from build123d import *

# Parameters (mm, degrees)
SHELL1_T           = -3
SKETCH2_R          = 35
CUT_EXTRUDE1_DEPTH = 131.048068171
SKETCH3_W          = 75
SKETCH3_H          = 50
CUT_EXTRUDE2_DEPTH = 131.048068171


with BuildPart() as part:
    # Sketch1 → Revolve1 (revolve)
    with BuildSketch(Plane.XY, mode=Mode.PRIVATE) as revolve1_sk:
        with BuildLine():
            Line((0, 40), (0, 0))
            Line((0, 0), (-87.5, 0))
            Line((-87.5, 0), (-87.5, 5))
            ThreePointArc((-87.5, 5), (-84.085301316, 16.215125476), (-75, 23.624343151))
            Line((-75, 23.624343151), (-35, 40))
            Line((-35, 40), (0, 40))
        make_face()
    revolve(revolve1_sk.sketch.rotate(Axis((0, 40, 0), (0, -1, 0)), 270), axis=Axis((0, 40, 0), (0, -1, 0)))

    # Shell1
    shell1_openings = [part.faces().sort_by_distance(p)[0] for p in [
        (0, 0, 0),
        (0, 40, 0),
    ]]
    offset(amount=SHELL1_T, openings=shell1_openings, kind=Kind.INTERSECTION)

    # Sketch2 → Cut-Extrude1 (cut, through all)
    with BuildSketch(Plane(origin=(0, 40, 0), x_dir=(1, 0, 0), z_dir=(0, 1, 0))):
        with Locations(Location((0, 0, 0), (0, 0, 180))):
            Circle(SKETCH2_R)
    extrude(amount=-CUT_EXTRUDE1_DEPTH, mode=Mode.SUBTRACT)

    # Sketch3 → Cut-Extrude2 (cut, through all)
    with BuildSketch(Plane(origin=(0, 0, 0), x_dir=(1, 0, 0), z_dir=(0, 1, 0))):
        with Locations((0, 87.5)):
            Rectangle(SKETCH3_W, SKETCH3_H)
    extrude(amount=CUT_EXTRUDE2_DEPTH, mode=Mode.SUBTRACT)


solid = part.part
The model under review builds one solid part; all positions refer to its coordinate system, in mm. A direction names the side the tool comes from. Coordinates: 2 decimals unless noted, no trailing zeros. Write each loop counter-clockwise with the first axis right and the second up, starting at its lowest first coordinate (ties: lowest second). Pieces come first, ordered by that corner, then holes. Notation, with made-up numbers: (15.5, -40) -> (29.5, -40) arc R16 cw to (29.5, -20) -> close; hole circle Ø9 at (20, 33). An arc over 180 degrees is marked (long way). Answer in a Markdown table with one row per item.
1. We need section C-C, the plane y = 13. State the section outline as (x, z) points.
Answers below:
| item | result |
|---|---|
| outline | (-37.5, -77.22) -> (-37.5, -73.5) arc R82.52 cw (long way) to (37.5, -73.5) -> (37.5, -77.22) arc R85.84 ccw (long way) to start |
2. We need section A-A, the plane z = 0. State the section outline as (x, y) points, and give its area (3 significant figures).
Answers below:
| item | result |
|---|---|
| outline | (-87.5, 0) -> (-84.5, 0) -> (-84.5, 5) arc R17.12 cw to (-73.86, 20.85) -> (-35, 36.76) -> (-35, 40) -> (-75, 23.62) arc R20.12 ccw to (-87.5, 5) -> close; (35, 36.76) -> (73.86, 20.85) arc R17.12 cw to (84.5, 5) -> (84.5, 0) -> (87.5, 0) -> (87.5, 5) arc R20.12 ccw to (75, 23.62) -> (35, 40) -> close |
| area | 418 mm^2 |
3. Wall thickness on probe 1 along X at (y, z) = (2.45, 0); probe 2 along X at (y, z) = (17.5, 29.5); probe 3 along Y at (x, z) = (-69, 45): over which ranges is each line inside the solid? List them lowest first. Write a range as [from, to].
Answers below:
| item | result |
|---|---|
| probe 1 | x = [-87.5, -84.5], [84.5, 87.5] |
| probe 2 | x = [-77.74, -73.37], [73.37, 77.74] |
| probe 3 | y = [13.26, 18.41] |
4. For faces 1 (the cylindrical face through (3.17, 2.54, 84.44)), 2 (the flat face through (-1, 26, -62.5)), 3 (the cylindrical face through (7.587, 38.402, -34.168)), list the 3-axis set-ups (+Z, -Z, +X, -X, +Y, -Y) from which the entire face can be reached by the end or side of a thin tool; tool diameter is ignored.
Answers below:
| item | result |
|---|---|
| face 1 | -Y |
| face 2 | -Z, +Y, -Y |
| face 3 | +Y, -Y |
5. Clearance check with flat-ended pins moving along their axes: pin 1 Ø8 at (x, y) = (-34, 18) entering from -Z; pin 2 Ø13 at (y, z) = (15.5, -68.5) entering from -X; pin 3 Ø8 at (x, y) = (-18, 25.5) entering from -Z. State where each tip first meets the part, or that it passes through.
Answers below:
| item | result |
|---|---|
| pin 1 | stops at z = -75.37 |
| pin 2 | stops at x = -58.9 |
| pin 3 | stops at z = -62.5 |
6. Draft analysis for pull direction X (two halves, no side actions). For faces 4 (the flat face through (37.5, 14, -73.2)), 5 (the cylindrical face through (3.305, 2.535, 87.438)), 6 (the flat face through (-65.2, 0, 54)), 7 (the flat face through (-37.5, 14, -73.2)), state which applies: +X half, -X half, draft (parallel to the pull), parting line (faces both ways), or undercut.
Answers below:
| item | result |
|---|---|
| face 4 | undercut |
| face 5 | parting line |
| face 6 | draft |
| face 7 | undercut |
7. We need section B-B, the plane x = 0. State the section outline as (y, z) points, and give its area (3 significant figures).
Answers below:
| item | result |
|---|---|
| outline | (0, 84.5) -> (5, 84.5) arc R17.12 cw to (20.85, 73.86) -> (36.76, 35) -> (40, 35) -> (23.62, 75) arc R20.12 ccw to (5, 87.5) -> (0, 87.5) -> close; (25.5, -62.5) -> (28.74, -62.5) -> (40, -35) -> (36.76, -35) -> close |
| area | 298 mm^2 |
